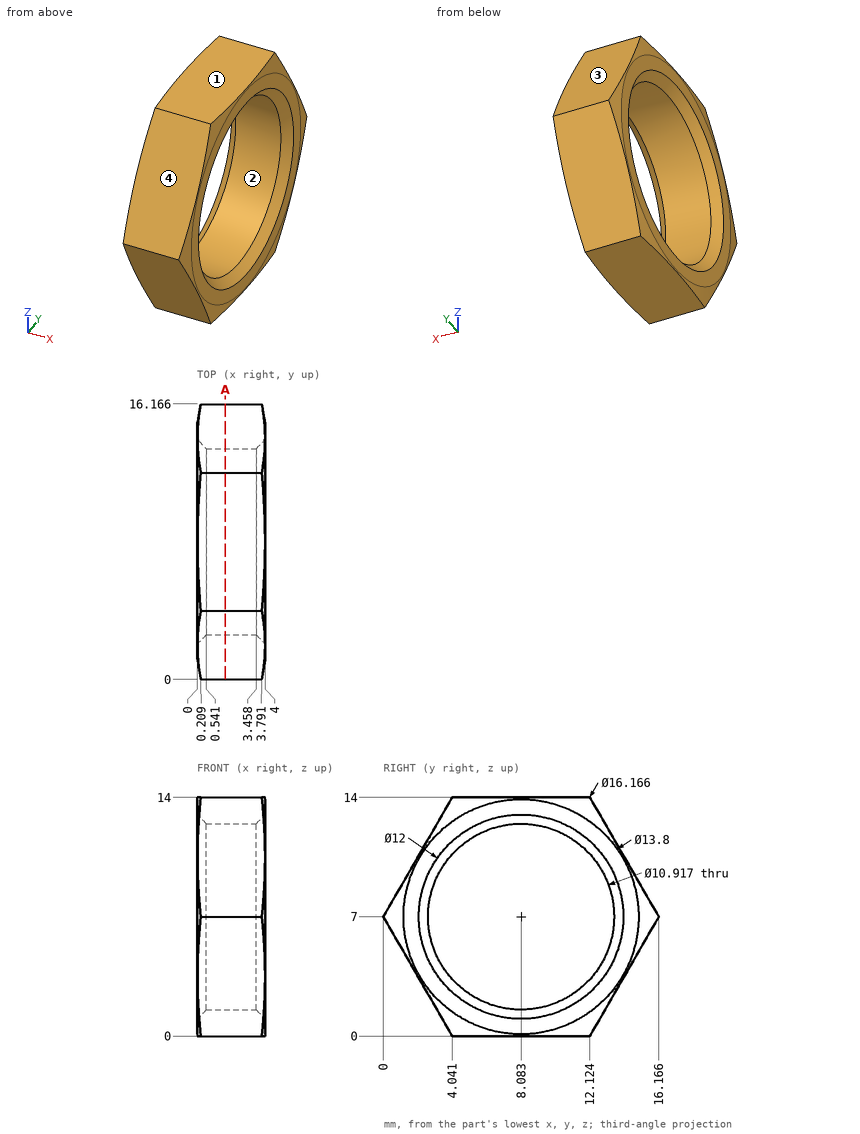
Here's the drawing with two shaded views (mm, measured from the low corner). I have some questions. Give positions to 0.01 mm unless a question says otherwise; leave off trailing zeros. Order: outer loops, then holes, each group sorted by start corner. A loop starts at its lowest first (then second) coordinate and runs counter-clockwise, first axis right, second up. Notation, with made-up numbers: M -38,-27 L -16,-27 A33 ccw -16,1 Z; hole C -10.75,-18 d2. An arc over 180 degrees is marked long. Answer as a JSON object with one key per item and string values. Group by question number.
1) Please list where these lines run through material, in increasing order: L1, parallel to Y at x = 1.9, z = 5.75 (1 decimal); L2, parallel to Z at x = 3.7, y = 4.5 (1 decimal); L3, parallel to Y at x = 3.75, z = 2 (1 decimal). Write a range as [from, to].
2) We'd pull the mould along Y, two halves only. Please class the marked faces 1, 2, 3 and 4: pulls with the +Y half, pulls with the -Y half, needs draft (parallel to the pull), parting line crosses it, or undercut.
3) I'm going to push a flat-ended pin straight in: pin 1 Ø1 at (x, z) = (1.5, 8.5) entering from -Y. Where does the tip first touch, or does it pass through?
4) Suppose I cut it at A-A, the plane x = 1.65. Write out the boundary of the cut face in (y, z) (1 decimal).
Results found:
{
 "1": {"L1": "[0.7, 2.8], [13.4, 15.4]", "L2": "[0, 2.6], [11.4, 14]", "L3": "[2.9, 5.2], [10.9, 13.3]"},
 "2": {"face 1": "needs draft", "face 2": "undercut", "face 3": "pulls with the +Y half", "face 4": "pulls with the -Y half"},
 "3": {"pin 1": "y = 0.58"},
 "4": {"outline": "M 0,7 L 4,0 L 12.1,0 L 16.2,7 L 12.1,14 L 4,14 Z; hole C 8.1,7 d10.9"}
}
